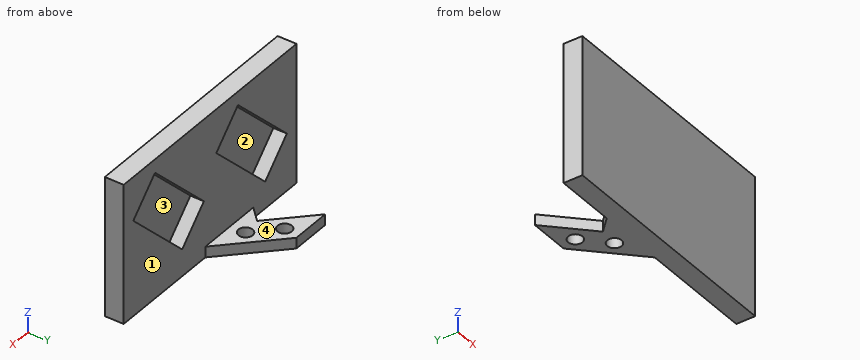
from build123d import *

# Parameters (mm, degrees)
SKETCH1_W           = 90
SKETCH1_H           = 51.769552622
BOSS_EXTRUDE1_DEPTH = 5
SKETCH5_R           = 2.65
BOSS_EXTRUDE2_DEPTH = 4
CHAMFER1_SIZE       = 10
CHAMFER1_SIZE2      = 7.071067812
SKETCH6_W           = 90
SKETCH6_H           = 51.769552622
BOSS_EXTRUDE3_DEPTH = 2


with BuildPart() as part:
    # Sketch1 → Boss-Extrude1 (new body)
    with BuildSketch(Plane(origin=(0, 0, 0), x_dir=(1, 0, 0), z_dir=(0, 1, 0))):
        with Locations((45, -25.884776311)):
            Rectangle(SKETCH1_W, SKETCH1_H)
        Polygon((5, -21.313708499), (30.455844123, -46.769552622), (41.769552622, -35.455844123), (16.313708499, -10), align=None, mode=Mode.SUBTRACT)
        Polygon((48.230447378, -21.313708499), (73.686291501, -46.769552622), (85, -35.455844123), (59.544155877, -10), align=None, mode=Mode.SUBTRACT)
    extrude(amount=BOSS_EXTRUDE1_DEPTH)

    # Sketch5 → Boss-Extrude2 (add)
    with BuildSketch(Plane(origin=(0, 0, 0), x_dir=(-1, 0, 0), z_dir=(0, 0, -1))):
        Polygon((-52.5, 0), (-27.751262658, 24.748737342), (-12.751262658, 24.748737342), (-37.5, 0), align=None)
        with Locations((-25.908116908, 19.091883092)):
            Circle(SKETCH5_R, mode=Mode.SUBTRACT)
        with Locations((-34.393398282, 10.606601718)):
            Circle(SKETCH5_R, mode=Mode.SUBTRACT)
    extrude(amount=-BOSS_EXTRUDE2_DEPTH)

    # Chamfer1
    chamfer1_edges = [part.edges().sort_by_distance(p)[0] for p in [
        (32.5, 5, 2),
    ]]
    chamfer1_side = [part.faces().sort_by_distance(p)[0] for p in [
        (45.087025644, 5, 25.465047734),
    ]]
    chamfer(chamfer1_edges, length=CHAMFER1_SIZE, length2=CHAMFER1_SIZE2, reference=chamfer1_side[0])

    # Sketch6 → Boss-Extrude3 (add)
    with BuildSketch(Plane.XZ):
        with Locations((45, 25.884776311)):
            Rectangle(SKETCH6_W, SKETCH6_H)
    extrude(amount=BOSS_EXTRUDE3_DEPTH)


solid = part.part
Work out the finished part from the listing and answer in its coordinate system (mm). Face numbers are marked on the shaded views. Give positions to 0.01 mm unless a question says otherwise; leave off trailing zeros. Loops run counter-clockwise (first coordinate to the right, second up) from the corner with the lowest first, then second, coordinate; pieces in that order, holes last. Notation, with made-up numbers: (88.25, 68) - (130.25, 68) arc R14 ccw to (130.25, 73) - close; hole circle Ø7 at (-31, 71.5). An arc over 180 degrees is marked (long way). Answer in a Markdown table with one row per item. Add a question column.
Q1. The part is cut by section D-D (y = 6.75). Determine the outline of the cut face in (x, z).
Q2. The part is cut by section B-B (x = 53). Determine the outline of the cut face in (y, z).
Q3. The part is cut by section A-A (y = 20.25). Determine the outline of the cut face in (x, z).
Q4. Each of these flat-tipped pins is pushed along its axis until it touches: P1, Ø1, axis at x = 41.5, y = 11, coming from the +Z side; P2, Ø3, axis at x = 49.5, z = 34.5, coming from the +Y side; P3, Ø4, axis at y = 21.5, z = 5.5, coming from the -X side; P4, Ø3, axis at x = 34.39, y = 10.61, coming from the -Z side. Where does it stop, or does it pass through?
Q5. The part is cut by section C-C (z = 6). Determine the outline of the cut face in (x, y), and give its area (3 significant figures).
Q6. Consider line 1 along X through (y, z) = (3.5, 44.5); line 2 along X through (y, z) = (2, 36); line 3 along Y through (x, z) = (66, 47.5). Determine where each line is inside the solid, lowest interval first.
Q7. Determine the mould class of the marked faces 1, 2, 3 and 4 for opening direction Z: released by +Z, released by -Z, zero draft, split by the parting line, or undercut.
Solution:
| question | item | result |
|---|---|---|
| 1 | outline | (24.25, 0) - (45.75, 0) - (45.75, 4) - (24.25, 4) - close |
| 2 | outline | (-2, 0) - (5, 0) - (5, 16.54) - (0, 16.54) - (0, 26.08) - (5, 26.08) - (5, 51.77) - (-2, 51.77) - close |
| 3 | outline | (17.25, 0) - (23.52, 0) - (23.52, 4) - (17.25, 4) - close; (28.29, 0) - (32.25, 0) - (32.25, 4) - (28.29, 4) - close |
| 4 | P1 | stops at z = 4 |
| 4 | P2 | stops at y = 5 |
| 4 | P3 | stops at x = 14.68 |
| 4 | P4 | passes through |
| 5 | outline | (0, -2) - (90, -2) - (90, 5) - (0, 5) - close |
| 5 | area | 630 mm² |
| 6 | line 1 | x = 0 to 28.19, 32.73 to 71.42, 75.96 to 90 |
| 6 | line 2 | x = 0 to 19.69, 41.23 to 62.92, 84.46 to 90 |
| 6 | line 3 | y = -2 to 5 |
| 7 | face 1 | zero draft |
| 7 | face 2 | undercut |
| 7 | face 3 | undercut |
| 7 | face 4 | released by +Z |
